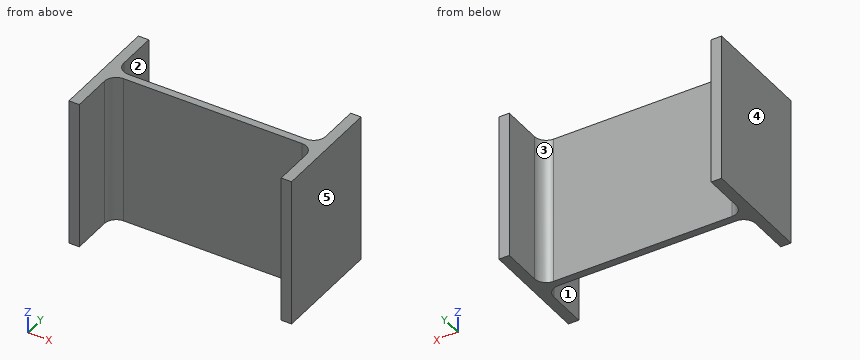
Autodesk Fusion 360 part; units mm, degrees
sketch "スケッチ1" plane through (0, 0, 0) normal (0, 0, 1) x (1, 0, 0)
  line L0 (0, 37.5) -> (0, -37.5)
  line L1 (150, -37.5) -> (150, 37.5)
  line L2 (143, -10.5) -> (143, -37.5)
  line L3 (7, -37.5) -> (7, -10.5)
  line L4 (0, -37.5) -> (7, -37.5)
  line L5 (143, -37.5) -> (150, -37.5)
  line L6 (135, 2.5) -> (15, 2.5)
  line L7 (15, -2.5) -> (135, -2.5)
  arc A0 (7, 10.5) -> (15, 2.5) centre (15, 10.5) ccw
  arc A1 (15, -2.5) -> (7, -10.5) centre (15, -10.5) ccw
  line L8 (7, 37.5) -> (0, 37.5)
  line L9 (7, 10.5) -> (7, 37.5)
  arc A2 (135, 2.5) -> (143, 10.5) centre (135, 10.5) ccw
  arc A3 (143, -10.5) -> (135, -2.5) centre (135, -10.5) ccw
  line L10 (143, 37.5) -> (143, 10.5)
  line L11 (150, 37.5) -> (143, 37.5)
extrude "押し出し1" add sketch "スケッチ1" along normal blind 100
CAD build for the part. Positions are in the model's coordinates, mm. Face numbers are marked on the shaded views. A direction names the side the tool comes from. Round coordinates to 2 decimals unless told otherwise and drop trailing zeros. Loops run counter-clockwise (first coordinate to the right, second up) from the corner with the lowest first, then second, coordinate; pieces in that order, holes last. Notation, with made-up numbers: M -4,54.5 L 43,54.5 A24 cw 43,71.5 Z; hole C -9,-31.5 d9. An arc over 180 degrees is marked long. Use a Markdown table: item, result. Add a question column.
(1) Which spindle directions (+Z, -Z, +X, -X, +Y, -Y) get a long thin tool onto all of the face, cutting with end or side? Do the marked faces 1 and 2. Say none if no direction does.
(2) Drill centre lines: line 1 (X direction, y = -19.5, z = 5); line 2 (Y direction, x = 104.5, z = 5); line 3 (X direction, y = 7, z = 28). Where is each one in solid material? Low to high.
(3) Cut at B-B (z = 54.5). Give the cut face in (x, y), and give its area (3 significant figures).
(4) Cut at A-A (y = -30). Give the cut face in (x, z), and give its area (3 significant figures).
(5) Flat gauge pins, fed straight in: pin 1 (5 mm diameter, centred on x = 117.5, z = 12.5, fed in from +Y); pin 2 (2 mm diameter, centred on x = 134.5, z = 82, fed in from -Y). Where does each tip first touch, or does it go through?
(6) Pull direction X, two halves, no side cores. Call the marked faces 3, 4 and 5: +X half, -X half, draft (parallel to the pull), parting line (faces both ways), or undercut.
(7) Cut at D-D (x = 75). Give the cut face in (y, z).
(8) Cut at C-C (y = 6.5). Give the cut face in (x, z), and give its area (3 significant figures).
Geometry says:
| question | item | result |
|---|---|---|
| 1 | face 1 | +Z, -Z, -Y |
| 1 | face 2 | +Z, -Z, +Y |
| 2 | line 1 | x = 0 to 7, 143 to 150 |
| 2 | line 2 | y = -2.5 to 2.5 |
| 2 | line 3 | x = 0 to 7.81, 142.19 to 150 |
| 3 | outline | M 0,-37.5 L 7,-37.5 L 7,-10.5 A8 cw 15,-2.5 L 135,-2.5 A8 cw 143,-10.5 L 143,-37.5 L 150,-37.5 L 150,37.5 L 143,37.5 L 143,10.5 A8 cw 135,2.5 L 15,2.5 A8 cw 7,10.5 L 7,37.5 L 0,37.5 Z |
| 3 | area | 1,780 mm² |
| 4 | outline | M 0,0 L 7,0 L 7,100 L 0,100 Z; M 143,0 L 150,0 L 150,100 L 143,100 Z |
| 4 | area | 1,400 mm² |
| 5 | pin 1 | stops at y = 2.5 |
| 5 | pin 2 | stops at y = -2.52 |
| 6 | face 3 | undercut |
| 6 | face 4 | -X half |
| 6 | face 5 | +X half |
| 7 | outline | M -2.5,0 L 2.5,0 L 2.5,100 L -2.5,100 Z |
| 8 | outline | M 0,0 L 8.07,0 L 8.07,100 L 0,100 Z; M 141.93,0 L 150,0 L 150,100 L 141.93,100 Z |
| 8 | area | 1,610 mm² |
